Source: CAD feature listing. Evaluate the final solid. Frame: model axes, mm. Face numbers are marked on the shaded views. A direction names the side the tool comes from. Round coordinates to 2 decimals unless told otherwise and drop trailing zeros. Loops run counter-clockwise (first coordinate to the right, second up) from the corner with the lowest first, then second, coordinate; pieces in that order, holes last.
Item 1: First-contact query: P1, Ø4, axis at y = -14, z = -267, coming from the -X side; P2, Ø5, axis at y = 0.5, z = -234, coming from the -X side; P3, Ø5, axis at y = -4.5, z = -46, coming from the +X side. Flat tips, straight axial feed; report the tip coordinate or a pass-through.
Item 2: Section query A-A on y = -4. Return loops of the section in (x, z).
Item 3: Section query C-C on z = -147.5. Return loops of the section in (x, y), then the cut area to 3 significant figures.
Item 4: Pull-direction query (X, two-part tool) for the marked faces 3, 4 and 5; classes: released by +X, released by -X, zero draft, split by the parting line, or undercut.
Item 5: Section query B-B on z = -91.5. Return loops of the section in (x, y), then the cut area to 3 significant figures.
Item 6: Access query for the marked faces 1 and 2. Directions: +Z, -Z, +X, -X, +Y, -Y. A direction counts if a zero-diameter tool reaches every point of the face in a straight line with its end or side. Return the directions, or none.
Item 7: Ray query, L1, parallel to X at y = 20.25, z = -300; L2, parallel to Z at x = -15.5, y = 18.5; L3, parallel to X at y = 18, z = 0. Return the intervals inside material, ascending.
```python
from build123d import *

# Parameters (mm, degrees)
SKETCH1_R             = 45
SKETCH1_R_2           = 22.5
BOSS_EXTRUDE1_DEPTH   = 31.65
SKETCH1_R_3           = 56.25
SKETCH1_R_4           = 28.15
BOSS_EXTRUDE1_2_DEPTH = 31.65
BOSS_EXTRUDE2_DEPTH   = 12.5
CUT_EXTRUDE1_DEPTH    = 5
CUT_EXTRUDE2_DEPTH    = 367.176207583
FILLET1_R             = 5


with BuildPart() as part:
    # Sketch1 → Boss-Extrude1 (new, symmetric)
    with BuildSketch(Plane(origin=(0, 0, 0), x_dir=(1, 0, 0), z_dir=(0, 1, 0))):
        with Locations(Location((0, 0, 0), (0, 0, 270))):
            Circle(SKETCH1_R)
        with Locations(Location((0, 0, 0), (0, 0, 270))):
            Circle(SKETCH1_R_2, mode=Mode.SUBTRACT)
    extrude(amount=BOSS_EXTRUDE1_DEPTH, both=True)



with BuildPart() as body_2:
    # Sketch1 → Boss-Extrude1 2 (new, symmetric)
    with BuildSketch(Plane(origin=(0, 0, 0), x_dir=(1, 0, 0), z_dir=(0, 1, 0))):
        with Locations(Location((0, 300, 0), (0, 0, 270))):
            Circle(SKETCH1_R_3)
        with Locations(Location((0, 300, 0), (0, 0, 270))):
            Circle(SKETCH1_R_4, mode=Mode.SUBTRACT)
    extrude(amount=BOSS_EXTRUDE1_2_DEPTH, both=True)


with BuildPart() as part_1:
    add(part.part)

    add(body_2.part)  # Boss-Extrude2 merges body 2
    # Sketch2 → Boss-Extrude2 (add, symmetric)
    with BuildSketch(Plane(origin=(0, 0, 0), x_dir=(1, 0, 0), z_dir=(0, 1, 0))):
        with BuildLine():
            Line((56.210435304, 297.890625), (44.968348244, -1.6875))
            ThreePointArc((44.968348244, -1.6875), (0, -45), (-44.968348244, -1.6875))
            Line((-44.968348244, -1.6875), (-56.210435304, 297.890625))
            ThreePointArc((-56.210435304, 297.890625), (0, 356.25), (56.210435304, 297.890625))
        make_face()
    extrude(amount=BOSS_EXTRUDE2_DEPTH, both=True)

    # Sketch3 → Cut-Extrude1 (cut)
    with BuildSketch(Plane(origin=(0, 12.5, 0), x_dir=(1, 0, 0), z_dir=(0, 1, 0))):
        with BuildLine():
            Line((22.255863805, 59.73892388), (28.619814412, 229.324907336))
            ThreePointArc((28.619814412, 229.324907336), (0, 223.75), (-28.619814412, 229.324907336))
            Line((-28.619814412, 229.324907336), (-22.255863805, 59.73892388))
            ThreePointArc((-22.255863805, 59.73892388), (0, 63.75), (22.255863805, 59.73892388))
        make_face()
    cut_extrude1 = extrude(amount=-CUT_EXTRUDE1_DEPTH, mode=Mode.SUBTRACT)

    # Mirror1: Cut-Extrude1 across plane
    add(cut_extrude1.mirror(Plane.ZX), mode=Mode.SUBTRACT)

    # Sketch4 → Cut-Extrude2 (cut, through all)
    with BuildSketch(Plane(origin=(0, 31.65, 0), x_dir=(1, 0, 0), z_dir=(0, 1, 0))):
        with BuildLine():
            Line((6.3, 272.564029086), (6.3, 264.864029086))
            Line((6.3, 264.864029086), (-6.3, 264.864029086))
            Line((-6.3, 264.864029086), (-6.3, 272.564029086))
            ThreePointArc((-6.3, 272.564029086), (0, 328.15), (6.3, 272.564029086))
        make_face()
    extrude(amount=-CUT_EXTRUDE2_DEPTH, mode=Mode.SUBTRACT)

    # Fillet1
    fillet1_edges = [part_1.edges().sort_by_distance(p)[0] for p in [
        (0, -31.65, -45),
        (0, -31.65, -356.25),
        (0, 31.65, -356.25),
        (0, 31.65, -45),
    ]]
    fillet(fillet1_edges, radius=FILLET1_R)


solid = part_1.part
```
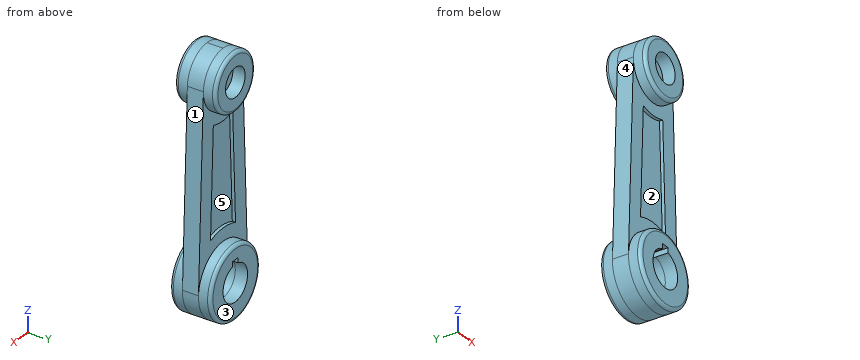
Data:
1. P1: stops at x = -55.1
1. P2: stops at x = -53.91
1. P3: stops at x = 46.85
2. outline: (-56.21, -297.89) arc R56.25 ccw (long way) to (56.21, -297.89) - (44.97, 1.69) arc R45 ccw to (-44.97, 1.69) - close; hole (-6.3, -272.56) arc R28.15 ccw (long way) to (6.3, -272.56) - (6.3, -264.86) - (-6.3, -264.86) - close
3. outline: (-50.57, -12.5) - (-25.55, -12.5) - (-25.55, -7.5) - (25.55, -7.5) - (25.55, -12.5) - (50.57, -12.5) - (50.57, 12.5) - (25.55, 12.5) - (25.55, 7.5) - (-25.55, 7.5) - (-25.55, 12.5) - (-50.57, 12.5) - close
3. area: 2,020 mm2
4. face 3: zero draft
4. face 4: released by -X
4. face 5: undercut
5. outline: (-48.47, -12.5) - (-23.45, -12.5) - (-23.45, -7.5) - (23.45, -7.5) - (23.45, -12.5) - (48.47, -12.5) - (48.47, 12.5) - (23.45, 12.5) - (23.45, 7.5) - (-23.45, 7.5) - (-23.45, 12.5) - (-48.47, 12.5) - close
5. area: 1,950 mm2
6. face 1: +Z, +X, +Y, -Y
6. face 2: -Y
7. L1: x = -56.25 to -28.15, 28.15 to 56.25
7. L2: z = -354.07 to -323.5, -276.5 to -245.93, -42.25 to -16.31, 16.31 to 42.25
7. L3: x = -45 to -22.5, 22.5 to 45
